The listing builds one solid part. Answer for the finished solid, in the listing's coordinates (mm). A direction names the side the tool comes from. Round coordinates to 2 decimals unless told otherwise and drop trailing zeros. Order: outer loops, then holes, each group sorted by start corner. A loop starts at its lowest first (then second) coordinate and runs counter-clockwise, first axis right, second up. Notation, with made-up numbers: M 56,65 L 100,65 A19 cw 100,99 Z; hole C -27,-13 d11. An arc over 180 degrees is marked long. Put each result on its own line as item: value. Start each with the question number.
1. Consider line 1 (X direction, y = 1.5, z = -13.5); line 2 (Z direction, x = 2.75, y = 1.8); line 3 (X direction, y = 1.05, z = -2.5). Determine where each line is inside the solid, lowest interval first.
2. Which of the six approach directions +Z, -Z, +X, -X, +Y, -Y give full straight-line access (tool end or side, diameter ignored) to faces 1 (the face through (-1.87, 1.41, -28.65)), 2 (the face through (10.8, 1, -10)), 3 (the face through (2.789, 1.014, -4.632))?
3. The part is cut by section C-C (z = -5). Give the vertices of the cut face in (x, y), then the cut area to 3 significant figures.
4. The part is cut by section D-D (x = 3). Give the vertices of the cut face in (y, z).
5. The mould has two halves that part along X. Classify faces 4 (the face through (2.868, 1.014, -10.289)), 5 (the face through (6.304, 1.392, -24.413)), 6 (the face through (0, 1, -28.8)), 7 (the face through (-2.789, 1.014, -10.368)): +X half, -X half, draft (parallel to the pull), parting line (faces both ways), or undercut.
6. The part is cut by section B-B (y = 0.4). Give the vertices of the cut face in (x, z).
7. The part is cut by section A-A (z = -17.5). Give the vertices of the cut face in (x, y).
from build123d import *

# Parameters (mm, degrees)
BOSS_EXTRUDE1_DEPTH = 2
FILLET1_R           = 1.9
BOSS_EXTRUDE2_DEPTH = 0.8
CUT_EXTRUDE1_REACH  = 35.153


with BuildPart() as part:
    # Sketch1 → Boss-Extrude1 (new body)
    with BuildSketch(Plane(origin=(0, 0, 0), x_dir=(1, 0, 0), z_dir=(0, 1, 0))):
        Polygon((-10.8, 0), (-10.8, 19.917157288), (-1.917157288, 28.8), (1.917157288, 28.8), (10.8, 19.917157288), (10.8, 0), align=None)
    extrude(amount=BOSS_EXTRUDE1_DEPTH)

    # Fillet1
    fillet1_edges = [part.edges().sort_by_distance(p)[0] for p in [
        (-10.8, 1, -19.917157288),
        (-1.917157288, 1, -28.8),
        (1.917157288, 1, -28.8),
        (10.8, 1, -19.917157288),
    ]]
    fillet(fillet1_edges, radius=FILLET1_R)

    # Sketch2 → Boss-Extrude2 (add)
    with BuildSketch(Plane.XZ):
        with BuildLine():
            Line((12.6, 0), (-12.6, 0))
            Line((-12.6, 0), (-12.6, -19.130151519))
            ThreePointArc((-12.6, -19.130151519), (-12.31835427, -20.546080219), (-11.51629509, -21.746446609))
            Line((-11.51629509, -21.746446609), (-3.746446609, -29.51629509))
            ThreePointArc((-3.746446609, -29.51629509), (-2.546080219, -30.31835427), (-1.130151519, -30.6))
            Line((-1.130151519, -30.6), (1.130151519, -30.6))
            ThreePointArc((1.130151519, -30.6), (2.546080219, -30.31835427), (3.746446609, -29.51629509))
            Line((3.746446609, -29.51629509), (11.51629509, -21.746446609))
            ThreePointArc((11.51629509, -21.746446609), (12.31835427, -20.546080219), (12.6, -19.130151519))
            Line((12.6, -19.130151519), (12.6, 0))
        make_face()
    extrude(amount=-BOSS_EXTRUDE2_DEPTH)

    # Sketch3 → Cut-Extrude1 (cut, up to next)
    with BuildSketch(Plane(origin=(0, 2, 0), x_dir=(1, 0, 0), z_dir=(0, 1, 0)), mode=Mode.PRIVATE) as cut_extrude1_sk1:
        Polygon((5.656854249, 7.5), (0, 13.156854249), (-5.656854249, 7.5), (0, 1.843145751), align=None)
    cut_extrude1_tool1 = extrude(cut_extrude1_sk1.sketch, amount=-CUT_EXTRUDE1_REACH, mode=Mode.PRIVATE) & part.part
    add(cut_extrude1_tool1.solids().sort_by_distance((0, 2, -7.5))[0], mode=Mode.SUBTRACT)


solid = part.part
Resolved:
1. line 1: -10.8 to 10.8
1. line 2: -27.97 to -10.41, -4.59 to 0
1. line 3: -10.8 to -0.66, 0.66 to 10.8
2. face 1: -Z, -X, +Y
2. face 2: +Z, -Z, +X, +Y
2. face 3: +Y, -Y
3. outline: M -12.6,0 L -3.16,0 L -3.16,2 L -10.8,2 L -10.8,0.8 L -12.6,0.8 Z; M 3.16,0 L 12.6,0 L 12.6,0.8 L 10.8,0.8 L 10.8,2 L 3.16,2 Z
3. area: 33.5 mm2
4. outline: M 0,-30.09 L 0.8,-30.09 L 0.8,-27.72 L 2,-27.72 L 2,-10.16 L 0,-10.16 Z; M 0,-4.84 L 2,-4.84 L 2,0 L 0,0 Z
5. face 4: undercut
5. face 5: +X half
5. face 6: draft
5. face 7: undercut
6. outline: M -12.6,-19.13 A3.7 ccw -11.52,-21.75 L -3.75,-29.52 A3.7 ccw -1.13,-30.6 L 1.13,-30.6 A3.7 ccw 3.75,-29.52 L 11.52,-21.75 A3.7 ccw 12.6,-19.13 L 12.6,0 L -12.6,0 Z; hole M -5.66,-7.5 L 0,-13.16 L 5.66,-7.5 L 0,-1.84 Z
7. outline: M -12.6,0 L 12.6,0 L 12.6,0.8 L 10.8,0.8 L 10.8,2 L -10.8,2 L -10.8,0.8 L -12.6,0.8 Z
